Check sheet for the drawn part. Datum: minimum x, y, z corner. Units: mm. Round coordinates to 2 decimals unless told otherwise and drop trailing zeros. Write each loop counter-clockwise with the first axis right and the second up, starting at its lowest first coordinate (ties: lowest second). Pieces come first, ordered by that corner, then holes. Notation, with made-up numbers: M 86.25,86.25 L 103.25,86.25 A21 ccw 103.25,90.25 Z; hole C -6,81.25 d6. An arc over 180 degrees is marked long. One line per item, written item: value. Start each with the question number.
1. Release check for a two-part mould opening along Z. For the marked faces 1, 2, 3 and 4 record: pulls with the +Z half, pulls with the -Z half, needs draft (parallel to the pull), parting line crosses it, or undercut.
2. Section check C-C (z = 8). Record the boundary of the cut face in (x, y).
3. Section check A-A (x = 2.5). Record the boundary of the cut face in (y, z), and give its area (3 significant figures).
4. Scan lines: probe 1 along X at (y, z) = (1.7, 7.5); probe 2 along X at (y, z) = (2.6, 3.75); probe 3 along Z at (x, y) = (6.75, 1.85). Record each from-to range of solid material in increasing order. Write a range as [from, to].
5. Section check D-D (x = 9.5). Record the boundary of the cut face in (y, z), and give its area (3 significant figures).
6. Section check B-B (y = 0.3). Record the boundary of the cut face in (x, z), and give its area (3 significant figures).
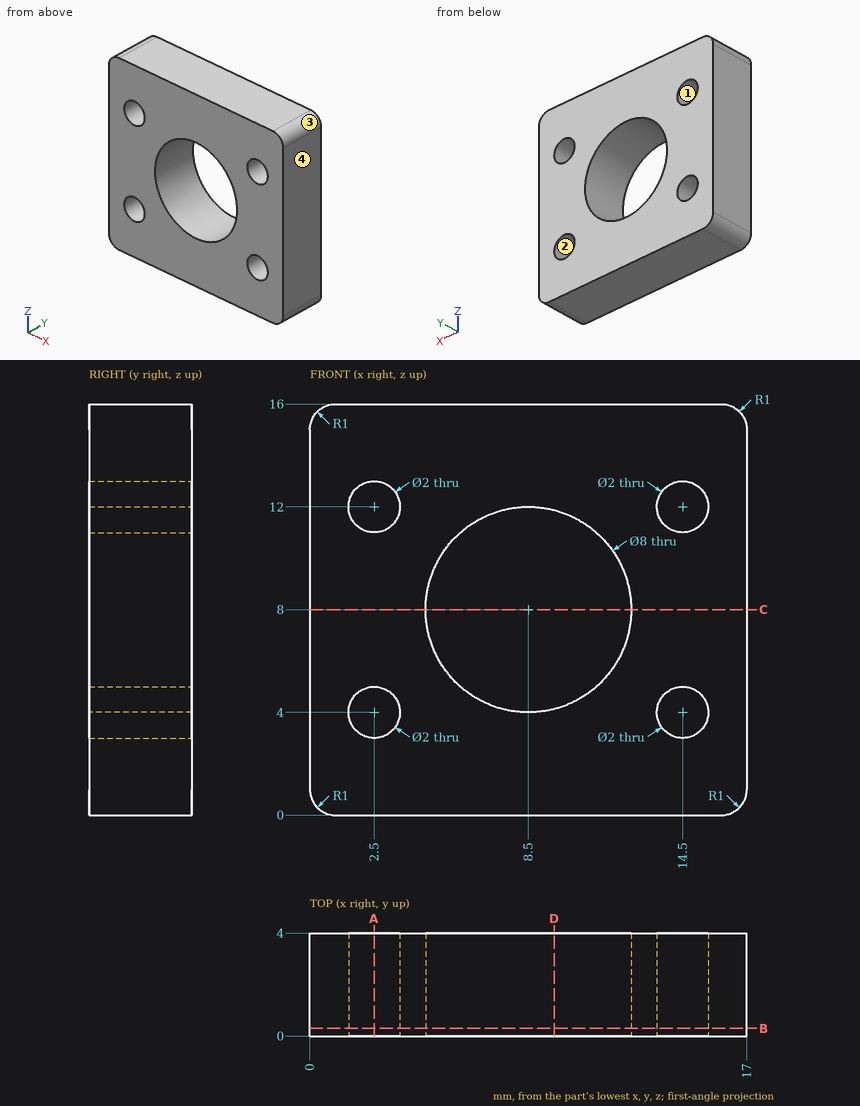
Result sheet:
1. face 1: undercut
1. face 2: undercut
1. face 3: pulls with the +Z half
1. face 4: needs draft
2. outline: M 0,0 L 4.5,0 L 4.5,4 L 0,4 Z; M 12.5,0 L 17,0 L 17,4 L 12.5,4 Z
3. outline: M 0,0 L 4,0 L 4,3 L 0,3 Z; M 0,5 L 4,5 L 4,11 L 0,11 Z; M 0,13 L 4,13 L 4,16 L 0,16 Z
3. area: 48.0 mm2
4. probe 1: x = [0, 4.53], [12.47, 17]
4. probe 2: x = [0, 1.53], [3.47, 13.53], [15.47, 17]
4. probe 3: z = [0, 4.4], [11.6, 16]
5. outline: M 0,0 L 4,0 L 4,4.13 L 0,4.13 Z; M 0,11.87 L 4,11.87 L 4,16 L 0,16 Z
5. area: 33.0 mm2
6. outline: M 0,1 A1 ccw 1,0 L 16,0 A1 ccw 17,1 L 17,15 A1 ccw 16,16 L 1,16 A1 ccw 0,15 Z; hole C 2.5,4 d2; hole C 2.5,12 d2; hole C 8.5,8 d8; hole C 14.5,4 d2; hole C 14.5,12 d2
6. area: 208 mm2
